```python
from build123d import *

# Parameters (mm, degrees)
F0_R     = 25.5
F0_R_2   = 23
F2_DEPTH = 25
F1_R     = 5
F1_R_2   = 1.5
F3_DEPTH = 14.5
F4_R     = 23
F4_R_2   = 5
F5_DEPTH = 3


with BuildPart() as f2:
    # F0 (on Top) → F2 (new body)
    with BuildSketch(Plane.XY):
        Circle(F0_R)
        Circle(F0_R_2, mode=Mode.SUBTRACT)
    extrude(amount=F2_DEPTH)



with BuildPart() as f3:
    # F1 (on Top) → F3 (new body)
    with BuildSketch(Plane.XY):
        Circle(F1_R)
        Circle(F1_R_2, mode=Mode.SUBTRACT)
    extrude(amount=F3_DEPTH)


with BuildPart() as f2_1:
    add(f2.part)

    add(f3.part)  # F5 merges F3
    # F4 (on face) → F5 (join)
    with BuildSketch(Plane.XY.offset(14.5)):
        Circle(F4_R)
        with BuildLine():
            ThreePointArc((19, 0), (15.723943, -5.346039), (9.473288, -4.854102))
            Line((9.473288, -4.854102), (7.543932, -7.509633))
            ThreePointArc((7.543932, -7.509633), (9.36326, -9.639792), (10.017221, -12.363735))
            ThreePointArc((10.017221, -12.363735), (3.078614, -18.289865), (-1.689118, -10.509633))
            Line((-1.689118, -10.509633), (-4.810882, -9.49531))
            ThreePointArc((-4.810882, -9.49531), (-15.371323, -11.16792), (-10.517221, -1.641208))
            Line((-10.517221, -1.641208), (-10.517221, 1.641208))
            ThreePointArc((-10.517221, 1.641208), (-15.371323, 11.16792), (-4.810882, 9.49531))
            Line((-4.810882, 9.49531), (-1.689118, 10.509633))
            ThreePointArc((-1.689118, 10.509633), (3.078614, 18.289865), (10.017221, 12.363735))
            ThreePointArc((10.017221, 12.363735), (9.36326, 9.639792), (7.543932, 7.509633))
            Line((7.543932, 7.509633), (9.473288, 4.854102))
            ThreePointArc((9.473288, 4.854102), (15.723943, 5.346039), (19, 0))
        make_face(mode=Mode.SUBTRACT)
        with BuildLine():
            Line((7.543932, -7.509633), (9.473288, -4.854102))
            ThreePointArc((9.473288, -4.854102), (7, 0), (9.473288, 4.854102))
            Line((9.473288, 4.854102), (7.543932, 7.509633))
            ThreePointArc((7.543932, 7.509633), (2.163119, 6.657396), (-1.689118, 10.509633))
            Line((-1.689118, 10.509633), (-4.810882, 9.49531))
            ThreePointArc((-4.810882, 9.49531), (-4.591091, 8.579815), (-4.517221, 7.641208))
            ThreePointArc((-4.517221, 7.641208), (-6.27458, 3.398568), (-10.517221, 1.641208))
            Line((-10.517221, 1.641208), (-10.517221, -1.641208))
            ThreePointArc((-10.517221, -1.641208), (-6.27458, -3.398568), (-4.517221, -7.641208))
            ThreePointArc((-4.517221, -7.641208), (-4.591091, -8.579815), (-4.810882, -9.49531))
            Line((-4.810882, -9.49531), (-1.689118, -10.509633))
            ThreePointArc((-1.689118, -10.509633), (2.163119, -6.657396), (7.543932, -7.509633))
        make_face()
        Circle(F4_R_2, mode=Mode.SUBTRACT)
    extrude(amount=-F5_DEPTH)


solid = f2_1.part
```
Work out the finished part from the listing and answer in its coordinate system (mm). A direction names the side the tool comes from. Give positions to 0.01 mm unless a question says otherwise; leave off trailing zeros. Write each loop counter-clockwise with the first axis right and the second up, starting at its lowest first coordinate (ties: lowest second). Pieces come first, ordered by that corner, then holes. Notation, with made-up numbers: (-18.5, 69.5) - (26.5, 69.5) arc R21 ccw to (26.5, 107.5) - close; hole circle Ø9 at (-30, 79). An arc over 180 degrees is marked (long way). Use one line per item in the form item = value.
1. A cutting plane is placed at B-B (y = -16). Write down the section's boundary in (x, z), and give its area (3 significant figures).
Filled in:
outline = (-19.86, 0) - (-16.52, 0) - (-16.52, 11.5) - (-0.76, 11.5) - (-0.76, 14.5) - (-16.52, 14.5) - (-16.52, 25) - (-19.86, 25) - close; (8.79, 11.5) - (16.52, 11.5) - (16.52, 0) - (19.86, 0) - (19.86, 25) - (16.52, 25) - (16.52, 14.5) - (8.79, 14.5) - close
area = 237 mm^2
2. A cutting plane is placed at C-C (x = 0). Write down the section's boundary in (y, z).
Filled in:
outline = (-25.5, 0) - (-23, 0) - (-23, 11.5) - (-16.82, 11.5) - (-16.82, 14.5) - (-23, 14.5) - (-23, 25) - (-25.5, 25) - close; (-7.91, 11.5) - (-5, 11.5) - (-5, 0) - (-1.5, 0) - (-1.5, 14.5) - (-7.91, 14.5) - close; (1.5, 0) - (5, 0) - (5, 11.5) - (7.91, 11.5) - (7.91, 14.5) - (1.5, 14.5) - close; (16.82, 11.5) - (23, 11.5) - (23, 0) - (25.5, 0) - (25.5, 25) - (23, 25) - (23, 14.5) - (16.82, 14.5) - close
3. Each of these flat-tipped pins is pushed along its axis until it touches: pin 1 Ø15.5 at (x, y) = (-10.52, 7.64) entering from -Z; pin 2 Ø10 at (y, z) = (14.5, 12) entering from -X; pin 3 Ø10 at (y, z) = (12, 14.5) entering from -X. Where does it stop, or does it pass through?
Filled in:
pin_1 = 11.5
pin_2 = -23.66
pin_3 = -24.52
4. A cutting plane is placed at D-D (x = -9). Write down the section's boundary in (y, z), and give its area (3 significant figures).
Filled in:
outline = (-23.86, 0) - (-21.17, 0) - (-21.17, 11.5) - (-13.45, 11.5) - (-13.45, 14.5) - (-21.17, 14.5) - (-21.17, 25) - (-23.86, 25) - close; (-1.84, 11.5) - (1.84, 11.5) - (1.84, 14.5) - (-1.84, 14.5) - close; (13.45, 11.5) - (21.17, 11.5) - (21.17, 0) - (23.86, 0) - (23.86, 25) - (21.17, 25) - (21.17, 14.5) - (13.45, 14.5) - close
area = 192 mm^2
5. For faces 4 (the face through (-1.2, 1.2, 0)), 5 (the face through (5, -5, 11.5)), 6 (the face through (-2.994, 22.804, 19.676)), determine the directions among +Z, -Z, +X, -X, +Y, -Y from which every point of the face is accessible in a straight line to the end or side of a thin tool.
Filled in:
face_4 = -Z, +X, -X, +Y, -Y
face_5 = -Z
face_6 = +Z
6. Determine the mould class of faces 1 (the face through (-2.994, 22.804, 5.67)), 2 (the face through (-4, 23, 0)), 3 (the face through (-5.5, -24.9, 12.3)) for opening direction Y: released by +Y, released by -Y, zero draft, split by the parting line, or undercut.
Filled in:
face_1 = undercut
face_2 = zero draft
face_3 = split by the parting line
7. Consider L1, parallel to Y at x = 0, z = 3.25; L2, parallel to X at y = 1, z = 9.75; L3, parallel to Y at x = 2, z = 12. Determine where each line is inside the solid, lowest interval first.
Filled in:
L1 = -25.5 to -23, -5 to -1.5, 1.5 to 5, 23 to 25.5
L2 = -25.48 to -22.98, -4.9 to -1.12, 1.12 to 4.9, 22.98 to 25.48
L3 = -25.42 to -18.01, -6.71 to 6.71, 18.01 to 25.42
8. A cutting plane is placed at A-A (z = 2.75). Write down the section's boundary in (x, y), and give its area (3 significant figures).
Filled in:
outline = circle Ø51 at (0, 0); circle Ø10 at (0, 0); hole circle Ø46 at (0, 0); hole circle Ø3 at (0, 0)
area = 452 mm^2
